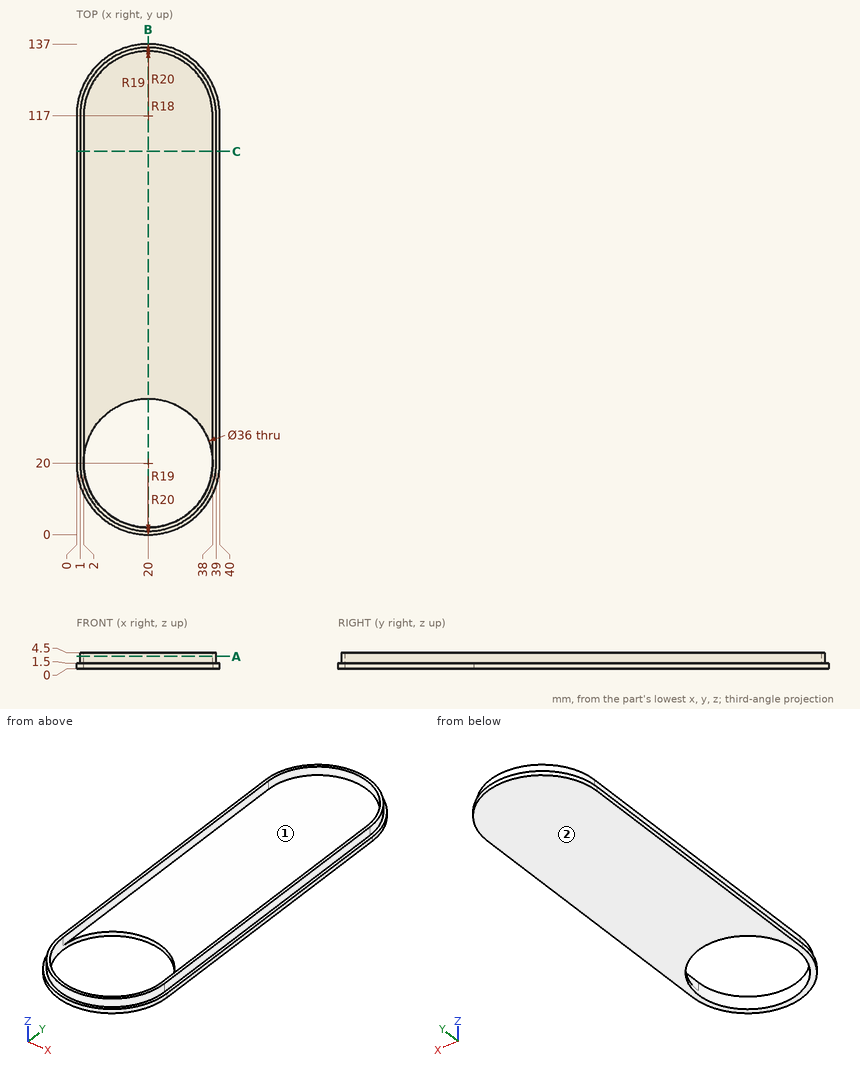
Here's the drawing with two shaded views (mm, measured from the low corner). I have some questions. Coordinates: 2 decimals unless noted, no trailing zeros. Write each loop counter-clockwise with the first axis right and the second up, starting at its lowest first coordinate (ties: lowest second). Pieces come first, ordered by that corner, then holes. Notation, with made-up numbers: (32, 48) -> (89, 48) arc R26 ccw to (89, 81) -> close; hole circle Ø10 at (54, 48.5). An arc over 180 degrees is marked (long way). Answer as CSV lines item,"result".
1) If we mould it in two halves opening along Y, with no side actions, what happens to the marked faces 1 and 2? For each: +Y half, -Y half, draft (parallel to the pull), parting line (faces both ways), or undercut.
Check result:
face 1,"undercut"
face 2,"draft"
2) If we section it at B-B on x = 20: Please give me the cut outline in (y, z).
Check result:
outline,"(0, 0) -> (2, 0) -> (2, 4.5) -> (1, 4.5) -> (1, 1.5) -> (0, 1.5) -> close; (38, 0) -> (137, 0) -> (137, 1.5) -> (136, 1.5) -> (136, 4.5) -> (135, 4.5) -> (135, 1.5) -> (38, 1.5) -> close"
3) If I drill on line 1 (Y direction, x = 20, z = 3.05); line 2 (X direction, y = 93.5, z = 2.65); line 3 (X direction, y = 20, z = 1.3), over which ranges is the centre line in solid material (lowest first)? Write a range as from..to.
Check result:
line 1,"1..2, 135..136"
line 2,"1..2, 38..39"
line 3,"0..2, 38..40"
4) If we section it at C-C on y = 107: Please give me the cut outline in (x, z).
Check result:
outline,"(0, 0) -> (40, 0) -> (40, 1.5) -> (39, 1.5) -> (39, 4.5) -> (38, 4.5) -> (38, 1.5) -> (2, 1.5) -> (2, 4.5) -> (1, 4.5) -> (1, 1.5) -> (0, 1.5) -> close"
5) If we section it at A-A on z = 3.5: Please give me the cut outline in (x, y), then the cut area to 3 significant figures.
Check result:
outline,"(1, 20) arc R19 ccw to (39, 20) -> (39, 117) arc R19 ccw to (1, 117) -> close; hole (2, 20) arc R18 ccw to (38, 20) -> (38, 117) arc R18 ccw to (2, 117) -> close"
area,"310 mm²"
6) Will these pins go through, and if not, where does the flat tip stop? P1, Ø0.9, axis at y = 68, z = 3.5, coming from the -X side; P2, Ø1, axis at x = 9.5, z = 1.5, coming from the +Y side; P3, Ø12, axis at x = 11, y = 103, coming from the +Z side.
Check result:
P1,"x = 1"
P2,"y = 134.32"
P3,"z = 1.5"
